```python
from build123d import *

# Parameters (mm, degrees)
BOSS_EXTRUDE3_DEPTH = 30
SKETCH6_R           = 11
SKETCH6_R_2         = 7
BOSS_EXTRUDE4_DEPTH = 12
CUT_EXTRUDE1_START  = -20
SKETCH7_R           = 7
CUT_EXTRUDE1_DEPTH  = 20


with BuildPart() as part:
    # Sketch3 → Boss-Extrude3 (new body)
    with BuildSketch(Plane.XY):
        Polygon((0, 8), (35, 8), (35, 66), (75, 66), (75, 58), (43, 58), (43, 0), (0, 0), align=None)
    extrude(amount=-BOSS_EXTRUDE3_DEPTH)

    # Sketch6 → Boss-Extrude4 (add)
    with BuildSketch(Plane(origin=(0, 66, 0), x_dir=(1, 0, 0), z_dir=(0, 1, 0))):
        with Locations(Location((60, 15, 0), (0, 0, 90))):
            Circle(SKETCH6_R)
        with Locations(Location((60, 15, 0), (0, 0, 270))):
            Circle(SKETCH6_R_2, mode=Mode.SUBTRACT)
    extrude(amount=BOSS_EXTRUDE4_DEPTH)

    # Sketch7 → Cut-Extrude1 (cut)
    with BuildSketch(Plane(origin=(0, 66, 0), x_dir=(1, 0, 0), z_dir=(0, 1, 0)).offset(CUT_EXTRUDE1_START)):
        with Locations(Location((60, 15, 0), (0, 0, 90))):
            Circle(SKETCH7_R)
    extrude(amount=CUT_EXTRUDE1_DEPTH, mode=Mode.SUBTRACT)


solid = part.part
```
Here's how the part is built. I have some questions about the finished solid (model axes, mm). A direction names the side the tool comes from. Round coordinates to 2 decimals unless told otherwise and drop trailing zeros. Write each loop counter-clockwise with the first axis right and the second up, starting at its lowest first coordinate (ties: lowest second). Pieces come first, ordered by that corner, then holes.
Q1. Will these pins go through, and if not, where does the flat tip stop? P1, Ø2, axis at y = 43.5, z = -16, coming from the -X side; P2, Ø3, axis at y = 49.5, z = -22.5, coming from the +X side; P3, Ø18, axis at x = 60, z = -15, coming from the -Y side.
Q2. If we section it at D-D on y = 11.5: Write out the boundary of the cut face in (x, z).
Q3. Please list where these lines run through material, in increasing order: probe 1 along Z at (x, y) = (60, 67); probe 2 along X at (y, z) = (65.5, -15); probe 3 along X at (y, z) = (70.75, -15).
Q4. If we mould it in two halves opening along X, with no side actions, what happens to faces 4 (the flat face through (75, 62, -15)), 5 (the flat face through (46, 66, -15)), 6 (the cylindrical face through (53, 66, -15)), 7 (the cylindrical face through (49.094, 71.916, -13.568))? For each: +X half, -X half, draft (parallel to the pull), parting line (faces both ways), or undercut.
Q5. If we section it at B-B on z = -15: Write out the boundary of the cut face in (x, y).
Q6. Which directions (+Z, -Z, +X, -X, +Y, -Y) give clear straight access to the entire face, cutting with the end or side of a thin tool? Please do faces 1 (the flat face through (52, 58, -15)), 2 (the flat face through (22, 0, -15)), 3 (the flat face through (35, 37, -15)).
Q7. If we section it at C-C on z = -2.5: Write out the boundary of the cut face in (x, y), plus the area to 3 significant figures.
Q8. If we section it at A-A on x = 60: Write out the boundary of the cut face in (y, z), plus the area to 3 significant figures.
Answer below:
1. P1: stops at x = 35
1. P2: stops at x = 43
1. P3: stops at y = 58
2. outline: (35, -30) - (43, -30) - (43, 0) - (35, 0) - close
3. probe 1: z = -26 to -22, -8 to -4
3. probe 2: x = 35 to 53, 67 to 75
3. probe 3: x = 49 to 53, 67 to 71
4. face 4: +X half
4. face 5: draft
4. face 6: undercut
4. face 7: parting line
5. outline: (0, 0) - (43, 0) - (43, 58) - (53, 58) - (53, 78) - (49, 78) - (49, 66) - (35, 66) - (35, 8) - (0, 8) - close; (67, 58) - (75, 58) - (75, 66) - (71, 66) - (71, 78) - (67, 78) - close
6. face 1: +Z, -Z, +X, -Y
6. face 2: +Z, -Z, +X, -X, -Y
6. face 3: +Z, -Z, -X, +Y
7. outline: (0, 0) - (43, 0) - (43, 58) - (75, 58) - (75, 66) - (35, 66) - (35, 8) - (0, 8) - close
7. area: 1,060 mm2
8. outline: (58, -30) - (66, -30) - (66, -26) - (78, -26) - (78, -22) - (58, -22) - close; (58, -8) - (78, -8) - (78, -4) - (66, -4) - (66, 0) - (58, 0) - close
8. area: 224 mm2
